Geometry: final body of the model. Coordinates: model frame, mm. Face numbers are marked on the shaded views. A direction names the side the tool comes from. Give positions to 0.01 mm unless a question says otherwise; leave off trailing zeros. Order: outer loops, then holes, each group sorted by start corner. A loop starts at its lowest first (then second) coordinate and runs counter-clockwise, first axis right, second up. Notation, with made-up numbers: (67.5, 32) -> (82.5, 32) arc R31 cw to (82.5, 59) -> close; hole circle Ø4 at (72.5, 8). An arc over 180 degrees is marked (long way). Write item = value, one per line.
```python
from build123d import *

# Parameters (mm, degrees)
F1_DEPTH      = 41
F3_DEPTH      = 9
F4_SIZE       = 23.8
F5_SIZE       = 23.8
F7_DEPTH      = 9
F9_DEPTH      = 28.2
F11_DEPTH     = 34.5
F13_DEPTH     = 32.2
F14_R         = 4.49999
F15_T4_DEPTH  = 56.311183182
F15_T10_DEPTH = 35.158116908
F15_T15_DEPTH = 56.311183182
F15_T21_DEPTH = 35.158116908
F15_T23_DEPTH = 61.25
F15_T25_DEPTH = 37.45
F15_T28_ANGLE = 90
F15_T30_ANGLE = 90
F15_T32_ANGLE = 90


# Not quite as in the source:
# - a fillet or chamfer that OpenCascade refuses, or shapes differently, is made with other operations: its cross-section is extruded or revolved along the edge and cut away or added
# - a fillet or chamfer is up to 0.001 mm smaller than in the source, because OpenCascade refuses the exact size


with BuildPart() as f1:
    # F0 (on Top) → F1 (new body)
    with BuildSketch(Plane.XY):
        Polygon((0, 70), (0, 0), (70, 0), (70, 9), (9, 9), (9, 18), (70, 18), (70, 27), (46.091883092, 27), (70, 50.908116908), (63.6360389693, 57.2720779386), (33.3639610307, 27), (27, 33.3639610307), (57.2720779386, 63.6360389693), (50.908116908, 70), (27, 46.091883092), (27, 70), (18, 70), (18, 27), (9, 27), (9, 70), align=None)
    extrude(amount=F1_DEPTH)

    # F2 (on face) → F3 (join)
    with BuildSketch(Plane(origin=(0, 0, 0), x_dir=(1, 0, 0), z_dir=(0, 0, -1))):
        Polygon((70, -50.908116908), (70, 0), (0, 0), (0, -70), (50.908116908, -70), align=None)
    extrude(amount=F3_DEPTH)

    # F4
    f4_edges = [f1.edges().sort_by_distance(p)[0] for p in [
        (70, 4.5, 41),
        (70, 22.5, 41),
        (22.5, 70, 41),
        (4.5, 70, 41),
    ]]
    chamfer(f4_edges, length=F4_SIZE)

    # F5
    f5_edges = [f1.edges().sort_by_distance(p)[0] for p in [
        (66.818019, 54.090097, 41),
        (54.090097, 66.818019, 41),
    ]]
    chamfer(f5_edges, length=F5_SIZE)

    # F6 (on face) → F7 (cut, through all)
    with BuildSketch(Plane.XY):
        with BuildLine():
            Line((9, 56.5), (9, 31.5))
            ThreePointArc((9, 31.5), (10.3180194847, 28.3180194847), (13.5, 27))
            ThreePointArc((13.5, 27), (16.6819805153, 28.3180194847), (18, 31.5))
            Line((18, 31.5), (18, 56.5))
            ThreePointArc((18, 56.5), (16.6819805153, 59.6819805153), (13.5, 61))
            ThreePointArc((13.5, 61), (10.3180194847, 59.6819805153), (9, 56.5))
        make_face()
        with BuildLine():
            Line((56.5, 18), (13.5, 18))
            ThreePointArc((13.5, 18), (10.3180194847, 16.6819805153), (9, 13.5))
            ThreePointArc((9, 13.5), (10.3180194847, 10.3180194847), (13.5, 9))
            Line((13.5, 9), (56.5, 9))
            ThreePointArc((56.5, 9), (59.6819805153, 10.3180194847), (61, 13.5))
            ThreePointArc((61, 13.5), (59.6819805153, 16.6819805153), (56.5, 18))
        make_face()
        with BuildLine():
            Line((47.7261363926, 54.0900974233), (30.1819805153, 36.545941546))
            ThreePointArc((30.1819805153, 36.545941546), (28.8639610307, 33.3639610307), (30.1819805153, 30.1819805153))
            ThreePointArc((30.1819805153, 30.1819805153), (33.3639610307, 28.8639610307), (36.545941546, 30.1819805153))
            Line((36.545941546, 30.1819805153), (54.0900974233, 47.7261363926))
            ThreePointArc((54.0900974233, 47.7261363926), (55.408116908, 50.908116908), (54.0900974233, 54.0900974233))
            ThreePointArc((54.0900974233, 54.0900974233), (50.908116908, 55.408116908), (47.7261363926, 54.0900974233))
        make_face()
        Polygon((40.0441558773, 65.5), (31.5, 65.5), (31.5, 56.9558441227), align=None)
        Polygon((65.5, 40.0441558773), (56.9558441227, 31.5), (65.5, 31.5), align=None)
    extrude(amount=-F7_DEPTH, mode=Mode.SUBTRACT)

    # F8 (on face) → F9 (cut)
    with BuildSketch(Plane(origin=(9.545941546, -9.545941546, 0), x_dir=(0.7071067812, 0.7071067812, 0), z_dir=(0.7071067812, -0.7071067812, 0))):
        Polygon((56.1837661841, 32), (56.1837661841, 9), (76.4949493661, 9), (76.4949493661, 13.4720779386), (57.9670273048, 32), align=None)
    extrude(amount=-F9_DEPTH, mode=Mode.SUBTRACT)

    # F10 (on face) → F11 (cut)
    with BuildSketch(Plane.YZ.offset(27)):
        Polygon((50.591883092, 22.8801948466), (50.591883092, 9), (61, 9), (61, 13.4720779386), (51.591883092, 22.8801948466), align=None)
    extrude(amount=-F11_DEPTH, mode=Mode.SUBTRACT)

    # F12 (on face) → F13 (cut)
    with BuildSketch(Plane(origin=(0, 27, 0), x_dir=(-1, 0, 0), z_dir=(0, 1, 0))):
        Polygon((-61, 13.4720779386), (-61, 9), (-50.591883092, 9), (-50.591883092, 22.8801948466), (-51.591883092, 22.8801948466), align=None)
    extrude(amount=-F13_DEPTH, mode=Mode.SUBTRACT)

    # F14 (radius 4.5 in the source; OpenCascade refuses exactly that, so slightly less here)
    f14_edges = [f1.edges().sort_by_distance(p)[0] for p in [
        (35, 0, -9),
        (70, 25.454058, -9),
        (60.454058, 60.454058, -9),
        (25.454058, 70, -9),
        (0, 35, -9),
    ]]
    fillet(f14_edges, radius=F14_R)

    # F15: fillet of radius 4.5 on 7 edges, made by hand


with BuildPart() as f15_tool2:
    # F15_s3 → F15_t4 (new body)
    with BuildSketch(Plane(origin=(28.5909902577, 28.5909902577, 0), x_dir=(0, 0, 1), z_dir=(0.7071067812, 0.7071067812, 0))):
        with BuildLine():
            ThreePointArc((4.5, 13.5), (1.3180194847, 14.8180194847), (0, 18))
            Line((0, 18), (0, 13.5))
            Line((0, 13.5), (4.5, 13.5))
        make_face()
    extrude(amount=F15_T4_DEPTH)

    split(bisect_by=Plane.YZ.offset(70), keep=Keep.BOTTOM)

    split(bisect_by=Plane.XZ.offset(-18), keep=Keep.BOTTOM)


with BuildPart() as f1_1:
    add(f1.part)

    # F15_t1: union F15_tool2
    add(f15_tool2.part)


with BuildPart() as f15_tool8:
    # F15_s9 → F15_t10 (new body)
    with BuildSketch(Plane.YZ.offset(70)):
        with BuildLine():
            ThreePointArc((27, 4.5), (28.3180194847, 1.3180194847), (31.5, 0))
            Line((31.5, 0), (27, 0))
            Line((27, 0), (27, 4.5))
        make_face()
    extrude(amount=-F15_T10_DEPTH)

    split(bisect_by=Plane(origin=(9.545941546, -9.545941546, 0), x_dir=(0, 0, 1), z_dir=(0.7071067812, -0.7071067812, 0)), keep=Keep.TOP)


with BuildPart() as f1_2:
    add(f1_1.part)

    # F15_t7: union F15_tool8
    add(f15_tool8.part)


with BuildPart() as f15_tool13:
    # F15_s14 → F15_t15 (new body)
    with BuildSketch(Plane(origin=(68.4090097423, 68.4090097423, 0), x_dir=(0, 0, 1), z_dir=(-0.7071067812, -0.7071067812, 0))):
        with BuildLine():
            ThreePointArc((4.5, 13.5), (1.3180194847, 14.8180194847), (0, 18))
            Line((0, 18), (0, 13.5))
            Line((0, 13.5), (4.5, 13.5))
        make_face()
    extrude(amount=F15_T15_DEPTH)

    split(bisect_by=Plane.XZ.offset(-70), keep=Keep.TOP)

    split(bisect_by=Plane.YZ.offset(18), keep=Keep.TOP)


with BuildPart() as f1_3:
    add(f1_2.part)

    # F15_t12: union F15_tool13
    add(f15_tool13.part)


with BuildPart() as f15_tool19:
    # F15_s20 → F15_t21 (new body)
    with BuildSketch(Plane.XZ.offset(-34.841883092)):
        with BuildLine():
            ThreePointArc((27, 4.5), (28.3180194847, 1.3180194847), (31.5, 0))
            Line((31.5, 0), (27, 0))
            Line((27, 0), (27, 4.5))
        make_face()
    extrude(amount=-F15_T21_DEPTH)

    split(bisect_by=Plane(origin=(-3.1819805153, 3.1819805153, 0), x_dir=(0, 0, 1), z_dir=(-0.7071067812, 0.7071067812, 0)), keep=Keep.TOP)


with BuildPart() as f1_4:
    add(f1_3.part)

    # F15_t18: union F15_tool19
    add(f15_tool19.part)

    # F15_s24 → F15_t23 (cut)
    with BuildSketch(Plane.XY.offset(-9)):
        with BuildLine():
            ThreePointArc((0, 4.5), (1.3180194847, 1.3180194847), (4.5, 0))
            Line((4.5, 0), (0, 0))
            Line((0, 0), (0, 4.5))
        make_face()
    extrude(amount=F15_T23_DEPTH, mode=Mode.SUBTRACT)

    # F15_s26 → F15_t25 (cut)
    with BuildSketch(Plane.XY.offset(-9)):
        with BuildLine():
            ThreePointArc((70, 4.5), (68.6819805153, 1.3180194847), (65.5, 0))
            Line((65.5, 0), (70, 0))
            Line((70, 0), (70, 4.5))
        make_face()
        with BuildLine():
            ThreePointArc((0, 65.5), (1.3180194847, 68.6819805153), (4.5, 70))
            Line((4.5, 70), (0, 70))
            Line((0, 70), (0, 65.5))
        make_face()
    extrude(amount=F15_T25_DEPTH, mode=Mode.SUBTRACT)

    # F15_s27 → F15_t28 (revolve, cut)
    with BuildSketch(Plane.XZ.offset(-65.5)):
        with BuildLine():
            ThreePointArc((4.49999, -9), (1.3180165557, -7.6819834443), (0, -4.50001))
            Line((0, -4.50001), (0, -9))
            Line((0, -9), (4.49999, -9))
        make_face()
    revolve(axis=Axis((4.5, 65.5, -9), (0, 0, -1)), revolution_arc=F15_T28_ANGLE, mode=Mode.SUBTRACT)

    # F15_s29 → F15_t30 (revolve, cut)
    with BuildSketch(Plane.XZ.offset(-4.5)):
        with BuildLine():
            ThreePointArc((65.50001, -9), (68.6819834443, -7.6819834443), (70, -4.50001))
            Line((70, -4.50001), (70, -9))
            Line((70, -9), (65.50001, -9))
        make_face()
    revolve(axis=Axis((65.5, 4.5, -9), (0, 0, -1)), revolution_arc=F15_T30_ANGLE, mode=Mode.SUBTRACT)

    # F15_s31 → F15_t32 (revolve, cut)
    with BuildSketch(Plane.YZ.offset(4.5)):
        with BuildLine():
            ThreePointArc((4.49999, -9), (1.3180165557, -7.6819834443), (0, -4.50001))
            Line((0, -4.50001), (0, -9))
            Line((0, -9), (4.49999, -9))
        make_face()
    revolve(axis=Axis((4.5, 4.5, -9), (0, 0, -1)), revolution_arc=F15_T32_ANGLE, mode=Mode.SUBTRACT)


solid = f1_4.part
```
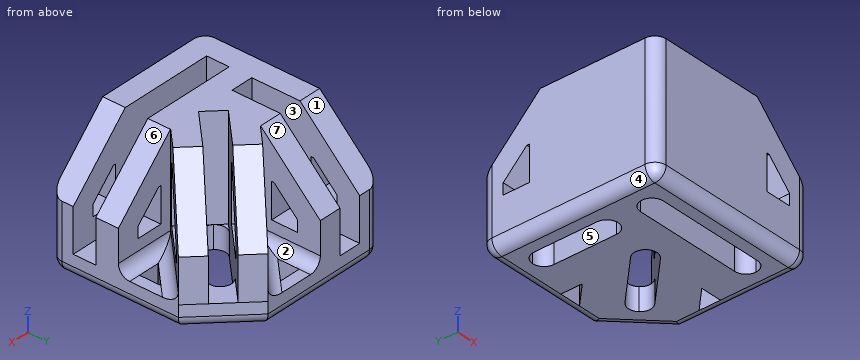
1) Section query A-A (x = 24.5). Output: boundary loops of the cut face in (y, z).
Check sheet entries:
outline = (0, -4.5) arc R4.5 ccw to (4.5, -9) -> (9, -9) -> (9, 41) -> (0, 41) -> close; (18, -9) -> (65.5, -9) arc R4.5 ccw to (70, -4.5) -> (70, 17.2) -> (46.2, 41) -> (18, 41) -> close; hole (50.59, 9) -> (61, 9) -> (61, 13.47) -> (51.59, 22.88) -> (50.59, 22.88) -> close
2) First-contact query: P1, Ø9.5, axis at x = 60.5, z = -6, coming from the +Y side; P2, Ø4.5, axis at x = 62, y = 14.5, coming from the +Z side; P3, Ø4.5, axis at x = 3.5, y = 53.5, coming from the +Z side. Flat tips, straight axial feed; report the tip coordinate or a pass-through.
Check sheet entries:
P1 = 65.02
P2 = 0
P3 = 35.95
3) Mould query, pull axis X, two halves, no side actions, for the marked faces 5, 6 and 7. Classes: +X half, -X half, draft (parallel to the pull), parting line (faces both ways), or undercut.
Check sheet entries:
face_5 = undercut
face_6 = +X half
face_7 = draft
4) Section query C-C (y = 16). Output: boundary loops of the cut face in (x, z), plus the area to 3 significant figures.
Check sheet entries:
outline = (0, -4.5) arc R4.5 ccw to (4.5, -9) -> (9.76, -9) -> (9.76, 0) -> (9, 0) -> (9, 41) -> (0, 41) -> close; (60.24, -9) -> (65.5, -9) arc R4.5 ccw to (70, -4.5) -> (70, 0) -> (60.24, 0) -> close
area = 536 mm²
5) Reachability of the marked faces 1, 2, 3 and 4 from +Z, -Z, +X, -X, +Y, -Y: full face, straight path, thin tool, end or side. Return the list, or none.
Check sheet entries:
face_1 = +Z, -X, +Y
face_2 = +Z, +Y
face_3 = +Z
face_4 = -Z, -X, +Y, -Y
6) Section query D-D (x = 17). Output: boundary loops of the cut face in (y, z), plus the area to 3 significant figures.
Check sheet entries:
outline = (0, -4.5) arc R4.5 ccw to (4.5, -9) -> (9, -9) -> (9, 41) -> (0, 41) -> close; (18, -9) -> (28.67, -9) -> (28.67, 0) -> (27, 0) -> (27, 41) -> (18, 41) -> close; (59.33, -9) -> (65.5, -9) arc R4.5 ccw to (70, -4.5) -> (70, 0) -> (59.33, 0) -> close
area = 1,000 mm²
7) Section query B-B (y = 25). Output: boundary loops of the cut face in (x, z).
Check sheet entries:
outline = (0, -4.5) arc R4.5 ccw to (4.5, -9) -> (65.5, -9) arc R4.5 ccw to (70, -4.5) -> (70, 17.2) -> (46.2, 41) -> (0, 41) -> close; hole (50.59, 9) -> (61, 9) -> (61, 13.47) -> (51.59, 22.88) -> (50.59, 22.88) -> close
8) Line query: line 1 (Y direction, x = 20, z = -1); line 2 (Y direction, x = 11, z = -6); line 3 (Y direction, x = 31, z = 11.5). Output: solid intervals per line, ascending. Write a range as from..to.
Check sheet entries:
line_1 = 0..9, 18..70
line_2 = 0.26..9.76, 17.24..27.76, 60.24..69.74
line_3 = 0..9, 18..29.36, 37.36..48.46
